Geometry check sheet. Reference: drawing and pictorial views, mm from the part's lowest x, y, z. A direction names the side the tool comes from. Round coordinates to 2 decimals unless told otherwise and drop trailing zeros. Write each loop counter-clockwise with the first axis right and the second up, starting at its lowest first coordinate (ties: lowest second). Pieces come first, ordered by that corner, then holes. Notation, with made-up numbers: M 65,81.5 L 104,81.5 A26 ccw 104,101.5 Z; hole C 11,41 d8. An arc over 180 degrees is marked long. One line per question, with ' | ' between items.
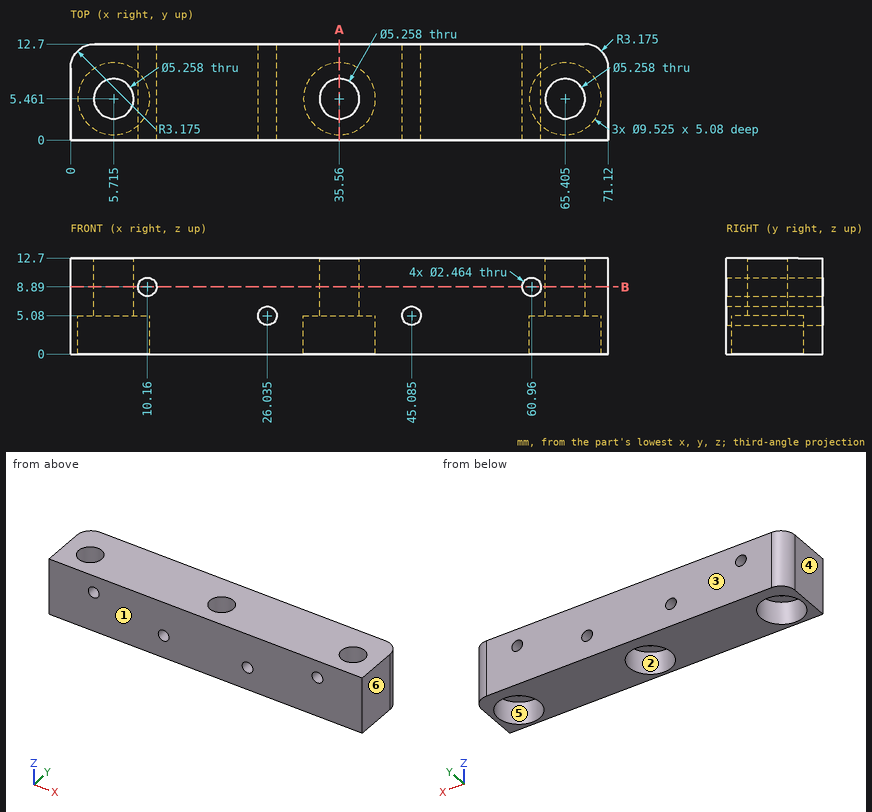
1. Tool access check on the marked faces 5 and 6. Record the directions out of +Z, -Z, +X, -X, +Y, -Y that give a thin tool (end or side, any length) a straight path to the whole face; none if there is none.
Results:
face 5: -Z | face 6: +Z, -Z, +X, +Y, -Y
2. Go/stop test with a flat-tipped pin: P1, Ø7, axis at x = 65.405, y = 5.461, coming from the -Z side. Record where the tip stops, or that it passes through.
Results:
P1: stops at z = 5.08
3. Thickness scan on line 1 (X direction, y = 5.5, z = 3.75); line 2 (X direction, y = 2.75, z = 4) (1 decimal); line 3 (X direction, y = 6.25, z = 2). Record the ranges inside material, lowest first.
Results:
line 1: x = 0 to 0.95, 10.48 to 30.8, 40.32 to 60.64, 70.17 to 71.12 | line 2: x = 0 to 1.8, 9.6 to 25.4, 26.6 to 31.6, 39.5 to 44.5, 45.7 to 61.5, 69.3 to 71.1 | line 3: x = 0 to 1.02, 10.41 to 30.86, 40.26 to 60.71, 70.1 to 71.12
4. Section check A-A, the plane x = 35.56. Record the cut outline in (y, z).
Results:
outline: M 0,0 L 0.7,0 L 0.7,5.08 L 2.83,5.08 L 2.83,12.7 L 0,12.7 Z; M 8.09,5.08 L 10.22,5.08 L 10.22,0 L 12.7,0 L 12.7,12.7 L 8.09,12.7 Z
5. Section check B-B, the plane z = 8.89. Count the separate pieces of the cut face and the enclosed holes in it, then the cut area to 3 significant figures.
Results:
separate pieces: 3 | enclosed holes: 3 | area: 771 mm2
6. Mould release check, pull along Y, two halves, no side actions. Record for the marked faces 1, 2, 3 and 4: pulls with the +Y half, pulls with the -Y half, needs draft (parallel to the pull), parting line crosses it, or undercut.
Results:
face 1: pulls with the -Y half | face 2: undercut | face 3: pulls with the +Y half | face 4: needs draft
